The model under review builds one solid part; all positions refer to its coordinate system, in mm. A direction names the side the tool comes from. Round coordinates to 2 decimals unless told otherwise and drop trailing zeros. Order: outer loops, then holes, each group sorted by start corner. A loop starts at its lowest first (then second) coordinate and runs counter-clockwise, first axis right, second up. Notation, with made-up numbers: M 80.25,-25 L 96.25,-25 A23 ccw 96.25,5 Z; hole C 18.25,69 d7. An arc over 180 degrees is marked long. Answer as a JSON object with one key per item and string values. Group by question number.
1) Insertion check: pin 1 Ø4 at (y, z) = (20.5, -59.5) entering from -X; pin 2 Ø6 at (x, z) = (18.5, -57) entering from -Y; pin 3 Ø20 at (x, z) = (32.5, 2.9) entering from +Y. Each pin has a flat end and moves straight along its axis. Give the tip position at first contact, or say it passes through.
2) The part is to be moulded in two halves that separate along Z. For faces 4 (the flat face through (-175, -2, 1)), 5 (the flat face through (-2, 2, 52.9)), 6 (the flat face through (-155, -2, -59)), say which applies: +Z half, -Z half, draft (parallel to the pull), parting line (faces both ways), or undercut.
3) To check wall thickness, follow line 1 (X direction, y = 135, z = 52); line 2 (Y direction, x = 160, z = 52); line 3 (Z direction, x = -25, y = 136). State the ranges of each line that lie inside material, in increasing order.
4) Consider section C-C, the plane z = 26. Write out the cut boundary in (x, y), then the cut area to 3 significant figures.
5) Consider section A-A, the plane x = -32.5. Write out the cut boundary in (y, z), then the cut area to 3 significant figures.
6) Consider section B-B, the plane y = -36. Write out the cut boundary in (x, z), then the cut area to 3 significant figures.
7) For faces 1 (the flat face through (2, -130, -59)), 2 (the flat face through (-2, -148.8, 1)), 3 (the cylindrical face through (48.984, 149.408, 3.625)), list the 3-axis set-ups (+Z, -Z, +X, -X, +Y, -Y) from which the entire face can be reached by the end or side of a thin tool; tool diameter is ignored.
8) Consider section D-D, the plane z = 7. Write out the cut boundary in (x, y), then the cut area to 3 significant figures.
```python
from build123d import *

# Parameters (mm, degrees)
SKETCH_1_W          = 350
SKETCH_1_H          = 300
EXTRUDE_1_DEPTH     = 52.9
SKETCH_2_W          = 310
SKETCH_2_H          = 260
EXTRUDE_2_DEPTH     = 12
SKETCH_6_W          = 310
SKETCH_6_H          = 260
EXTRUDE_3_DEPTH     = 4
EXTRUDE_3_DRAFT     = -45
SHELL_1_T           = -1.2
CUT_EXTRUDE_3_REACH = 262.692
SKETCH_12_R         = 3.5
CUT_EXTRUDE_4_REACH = 356.079
SKETCH_13_R         = 16.5


with BuildPart() as part:
    # 草图1 → 凸台-拉伸1 (new, symmetric)
    with BuildSketch(Plane.XY):
        Rectangle(SKETCH_1_W, SKETCH_1_H)
    extrude(amount=EXTRUDE_1_DEPTH, both=True)

    # 草图2 → 凸台-拉伸2 (add)
    with BuildSketch(Plane(origin=(0, 0, -52.9), x_dir=(-1, 0, 0), z_dir=(0, 0, -1))):
        Rectangle(SKETCH_2_W, SKETCH_2_H)
    extrude(amount=EXTRUDE_2_DEPTH)


with BuildPart() as extrude_3_tool:
    # 草图6 → 凸台-拉伸3 (with draft: the straight prism first)
    with BuildSketch(Plane(origin=(0, 0, -64.9), x_dir=(-1, 0, 0), z_dir=(0, 0, -1))):
        Rectangle(SKETCH_6_W, SKETCH_6_H)
    extrude(amount=EXTRUDE_3_DEPTH)
    # 凸台-拉伸3: the draft: its side faces are tilted about the plane it starts from
    extrude_3_sides = [extrude_3_tool.faces().sort_by_distance(p)[0] for p in [
        (155, 0, -66.9),
        (0, -130, -66.9),
        (-155, 0, -66.9),
        (0, 130, -66.9),
    ]]
    draft(extrude_3_sides, Plane(origin=(0, 0, -64.9), x_dir=(-1, 0, 0), z_dir=(0, 0, -1)), EXTRUDE_3_DRAFT)


with BuildPart() as part_1:
    add(part.part)

    # 凸台-拉伸3: add extrude_3_tool
    add(extrude_3_tool.part)

    # 抽壳1
    shell_1_openings = [part_1.faces().sort_by_distance(p)[0] for p in [
        (0, 0, -68.9),
    ]]
    offset(amount=SHELL_1_T, openings=shell_1_openings, kind=Kind.INTERSECTION)

    # 草图12 → 切除-拉伸3 (cut, up to next)
    with BuildSketch(Plane.XY.offset(52.9), mode=Mode.PRIVATE) as cut_extrude_3_sk1:
        with Locations((-160, 135)):
            Circle(SKETCH_12_R)
    cut_extrude_3_tool1 = extrude(cut_extrude_3_sk1.sketch, amount=-CUT_EXTRUDE_3_REACH, mode=Mode.PRIVATE) & part_1.part
    # 草图12 → 切除-拉伸3 (cut, up to next)
    with BuildSketch(Plane.XY.offset(52.9), mode=Mode.PRIVATE) as cut_extrude_3_sk2:
        with Locations((160, 135)):
            Circle(SKETCH_12_R)
    cut_extrude_3_tool2 = extrude(cut_extrude_3_sk2.sketch, amount=-CUT_EXTRUDE_3_REACH, mode=Mode.PRIVATE) & part_1.part
    # 草图12 → 切除-拉伸3 (cut, up to next)
    with BuildSketch(Plane.XY.offset(52.9), mode=Mode.PRIVATE) as cut_extrude_3_sk3:
        with Locations((160, -135)):
            Circle(SKETCH_12_R)
    cut_extrude_3_tool3 = extrude(cut_extrude_3_sk3.sketch, amount=-CUT_EXTRUDE_3_REACH, mode=Mode.PRIVATE) & part_1.part
    # 草图12 → 切除-拉伸3 (cut, up to next)
    with BuildSketch(Plane.XY.offset(52.9), mode=Mode.PRIVATE) as cut_extrude_3_sk4:
        with Locations((-160, -135)):
            Circle(SKETCH_12_R)
    cut_extrude_3_tool4 = extrude(cut_extrude_3_sk4.sketch, amount=-CUT_EXTRUDE_3_REACH, mode=Mode.PRIVATE) & part_1.part
    add(cut_extrude_3_tool1.solids().sort_by_distance((-160, 135, 52.9))[0], mode=Mode.SUBTRACT)
    add(cut_extrude_3_tool2.solids().sort_by_distance((160, 135, 52.9))[0], mode=Mode.SUBTRACT)
    add(cut_extrude_3_tool3.solids().sort_by_distance((160, -135, 52.9))[0], mode=Mode.SUBTRACT)
    add(cut_extrude_3_tool4.solids().sort_by_distance((-160, -135, 52.9))[0], mode=Mode.SUBTRACT)

    # 草图13 → 切除-拉伸4 (cut, up to next)
    with BuildSketch(Plane(origin=(0, 150, 0), x_dir=(1, 0, 0), z_dir=(0, 1, 0)), mode=Mode.PRIVATE) as cut_extrude_4_sk1:
        with Locations(Location((-32.5, -2.9, 0), (0, 0, 180))):
            Circle(SKETCH_13_R)
    cut_extrude_4_tool1 = extrude(cut_extrude_4_sk1.sketch, amount=-CUT_EXTRUDE_4_REACH, mode=Mode.PRIVATE) & part_1.part
    # 草图13 → 切除-拉伸4 (cut, up to next)
    with BuildSketch(Plane(origin=(0, 150, 0), x_dir=(1, 0, 0), z_dir=(0, 1, 0)), mode=Mode.PRIVATE) as cut_extrude_4_sk2:
        with Locations(Location((32.5, -2.9, 0), (0, 0, 180))):
            Circle(SKETCH_13_R)
    cut_extrude_4_tool2 = extrude(cut_extrude_4_sk2.sketch, amount=-CUT_EXTRUDE_4_REACH, mode=Mode.PRIVATE) & part_1.part
    # 草图13 → 切除-拉伸4 (cut, up to next)
    with BuildSketch(Plane(origin=(0, 150, 0), x_dir=(1, 0, 0), z_dir=(0, 1, 0)), mode=Mode.PRIVATE) as cut_extrude_4_sk3:
        with Locations(Location((97.5, -2.9, 0), (0, 0, 180))):
            Circle(SKETCH_13_R)
    cut_extrude_4_tool3 = extrude(cut_extrude_4_sk3.sketch, amount=-CUT_EXTRUDE_4_REACH, mode=Mode.PRIVATE) & part_1.part
    # 草图13 → 切除-拉伸4 (cut, up to next)
    with BuildSketch(Plane(origin=(0, 150, 0), x_dir=(1, 0, 0), z_dir=(0, 1, 0)), mode=Mode.PRIVATE) as cut_extrude_4_sk4:
        with Locations(Location((-97.5, -2.9, 0), (0, 0, 180))):
            Circle(SKETCH_13_R)
    cut_extrude_4_tool4 = extrude(cut_extrude_4_sk4.sketch, amount=-CUT_EXTRUDE_4_REACH, mode=Mode.PRIVATE) & part_1.part
    add(cut_extrude_4_tool1.solids().sort_by_distance((-32.5, 150, 2.9))[0], mode=Mode.SUBTRACT)
    add(cut_extrude_4_tool2.solids().sort_by_distance((32.5, 150, 2.9))[0], mode=Mode.SUBTRACT)
    add(cut_extrude_4_tool3.solids().sort_by_distance((97.5, 150, 2.9))[0], mode=Mode.SUBTRACT)
    add(cut_extrude_4_tool4.solids().sort_by_distance((-97.5, 150, 2.9))[0], mode=Mode.SUBTRACT)


solid = part_1.part
```
Results list:
{
 "1": {"pin 1": "x = -155", "pin 2": "y = -130", "pin 3": "y = -148.8"},
 "2": {"face 4": "draft", "face 5": "+Z half", "face 6": "undercut"},
 "3": {"line 1": "-175 to -163.5, -156.5 to 156.5, 163.5 to 175", "line 2": "-150 to -138.5, -131.5 to 131.5, 138.5 to 150", "line 3": "-52.9 to -51.7, 51.7 to 52.9"},
 "4": {"outline": "M -175,-150 L 175,-150 L 175,150 L -175,150 Z; hole M -173.8,-148.8 L 173.8,-148.8 L 173.8,148.8 L -173.8,148.8 Z", "area": "1,550 mm^2"},
 "5": {"outline": "M -150,-52.9 L -130,-52.9 L -130,-64.9 L -134,-68.9 L -132.3,-68.9 L -128.8,-65.4 L -128.8,-51.7 L -148.8,-51.7 L -148.8,51.7 L 148.8,51.7 L 148.8,19.4 L 150,19.4 L 150,52.9 L -150,52.9 Z; M 128.8,-65.4 L 132.3,-68.9 L 134,-68.9 L 130,-64.9 L 130,-52.9 L 150,-52.9 L 150,-13.6 L 148.8,-13.6 L 148.8,-51.7 L 128.8,-51.7 Z", "area": "662 mm^2"},
 "6": {"outline": "M -175,-52.9 L -155,-52.9 L -155,-64.9 L -159,-68.9 L -157.3,-68.9 L -153.8,-65.4 L -153.8,-51.7 L -173.8,-51.7 L -173.8,51.7 L 173.8,51.7 L 173.8,-51.7 L 153.8,-51.7 L 153.8,-65.4 L 157.3,-68.9 L 159,-68.9 L 155,-64.9 L 155,-52.9 L 175,-52.9 L 175,52.9 L -175,52.9 Z", "area": "761 mm^2"},
 "7": {"face 1": "+X, -X, -Y", "face 2": "none", "face 3": "+Y"},
 "8": {"outline": "M -175,-150 L 175,-150 L 175,150 L 113.48,150 L 113.48,148.8 L 173.8,148.8 L 173.8,-148.8 L -173.8,-148.8 L -173.8,148.8 L -113.48,148.8 L -113.48,150 L -175,150 Z; M -81.52,148.8 L -48.48,148.8 L -48.48,150 L -81.52,150 Z; M -16.52,148.8 L 16.52,148.8 L 16.52,150 L -16.52,150 Z; M 48.48,148.8 L 81.52,148.8 L 81.52,150 L 48.48,150 Z", "area": "1,400 mm^2"}
}
